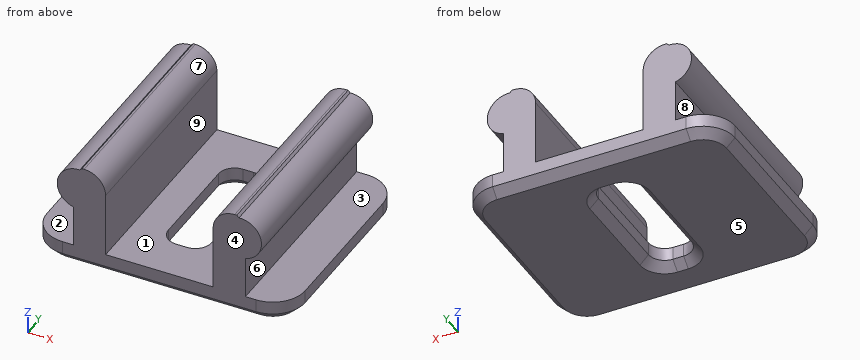
from build123d import *

# Parameters (mm, degrees)
BOX010_W                    = 2
BOX010_H                    = 6
BOX010_DEPTH                = 10
BOX008_W                    = 1.5
BOX008_H                    = 10
BOX008_DEPTH                = 5
CHAMFER004001002001005_SIZE = 0.4
CYLINDER004_R               = 1
CYLINDER004_DEPTH           = 10
CYLINDER003_R               = 1
CYLINDER003_DEPTH           = 10
BOX007_W                    = 12
BOX007_H                    = 10
BOX007_DEPTH                = 1
BOX009_W                    = 1.5
BOX009_H                    = 10
BOX009_DEPTH                = 5
CHAMFER004001002001006_SIZE = 0.4
FILLET_R                    = 0.75
FILLET001_R                 = 1.5
CHAMFER004001002001007_SIZE = 0.4
FILLET002_R                 = 1


with BuildPart() as cube010:
    # Box010 → Box010 (new body)
    with BuildSketch(Plane(origin=(-1, -3, 0), x_dir=(1, 0, 0), z_dir=(0, 0, 1))):
        with Locations((1, 3)):
            Rectangle(BOX010_W, BOX010_H)
    extrude(amount=BOX010_DEPTH)


with BuildPart() as chamfer004001002001005:
    # Box008 → Box008 (new body)
    with BuildSketch(Plane(origin=(-4, -5, 0), x_dir=(1, 0, 0), z_dir=(0, 0, 1))):
        with Locations((0.75, 5)):
            Rectangle(BOX008_W, BOX008_H)
    extrude(amount=BOX008_DEPTH)

    # Chamfer004001002001005
    chamfer004001002001005_edges = [chamfer004001002001005.edges().sort_by_distance(p)[0] for p in [
        (-4, 0, 5),
    ]]
    chamfer(chamfer004001002001005_edges, length=CHAMFER004001002001005_SIZE)


with BuildPart() as cylinder004:
    # Cylinder004 → Cylinder004 (new body)
    with BuildSketch(Plane(origin=(3.75, -5, 3.9), x_dir=(1, 0, 0), z_dir=(0, 1, 0))):
        Circle(CYLINDER004_R)
    extrude(amount=CYLINDER004_DEPTH)


with BuildPart() as cylinder003:
    # Cylinder003 → Cylinder003 (new body)
    with BuildSketch(Plane(origin=(-3.75, -5, 3.9), x_dir=(1, 0, 0), z_dir=(0, 1, 0))):
        Circle(CYLINDER003_R)
    extrude(amount=CYLINDER003_DEPTH)


with BuildPart() as cube007:
    # Box007 → Box007 (new body)
    with BuildSketch(Plane(origin=(-6, -5, 0), x_dir=(1, 0, 0), z_dir=(0, 0, 1))):
        with Locations((6, 5)):
            Rectangle(BOX007_W, BOX007_H)
    extrude(amount=BOX007_DEPTH)


with BuildPart() as cable_clip:
    # Box009 → Box009 (new body)
    with BuildSketch(Plane(origin=(2.5, -5, 0), x_dir=(1, 0, 0), z_dir=(0, 0, 1))):
        with Locations((0.75, 5)):
            Rectangle(BOX009_W, BOX009_H)
    extrude(amount=BOX009_DEPTH)

    # Chamfer004001002001006
    chamfer004001002001006_edges = [cable_clip.edges().sort_by_distance(p)[0] for p in [
        (4, 0, 5),
    ]]
    chamfer(chamfer004001002001006_edges, length=CHAMFER004001002001006_SIZE)

    # Fusion002: union Chamfer004001002001005, Cylinder004, Cylinder003, Cube007
    add(chamfer004001002001005.part)
    add(cylinder004.part)
    add(cylinder003.part)
    add(cube007.part)

    # Cut002008023012009006003002007003001002002: cut Cube010
    add(cube010.part, mode=Mode.SUBTRACT)

    # Fillet
    fillet_edges = [cable_clip.edges().sort_by_distance(p)[0] for p in [
        (1, -3, 0.5),
        (-1, -3, 0.5),
        (1, 3, 0.5),
        (-1, 3, 0.5),
    ]]
    fillet(fillet_edges, radius=FILLET_R)

    # Fillet001
    fillet001_edges = [cable_clip.edges().sort_by_distance(p)[0] for p in [
        (6, 5, 0.5),
        (-6, 5, 0.5),
        (6, -5, 0.5),
        (-6, -5, 0.5),
    ]]
    fillet(fillet001_edges, radius=FILLET001_R)

    # Chamfer004001002001007
    chamfer004001002001007_edges = [cable_clip.edges().sort_by_distance(p)[0] for p in [
        (4.25, -5, 0),
        (5.56066, -4.56066, 0),
        (6, 0, 0),
        (5.56066, 4.56066, 0),
        (3.25, 5, 0),
        (3.25, -5, 0),
        (0, 5, 0),
        (-1, 0, 0),
        (-0.78033, 2.78033, 0),
        (0, 3, 0),
        (0.78033, 2.78033, 0),
        (1, 0, 0),
        (0.78033, -2.78033, 0),
        (0, -3, 0),
        (-0.78033, -2.78033, 0),
        (0, -5, 0),
        (-3.25, 5, 0),
        (-3.25, -5, 0),
        (-4.25, 5, 0),
        (-5.56066, 4.56066, 0),
        (-6, 0, 0),
        (-5.56066, -4.56066, 0),
        (-4.25, -5, 0),
    ]]
    chamfer(chamfer004001002001007_edges, length=CHAMFER004001002001007_SIZE)

    # Fillet002
    fillet002_edges = [cable_clip.edges().sort_by_distance(p)[0] for p in [
        (2.5, 0, 5),
        (-2.5, 0, 5),
    ]]
    fillet(fillet002_edges, radius=FILLET002_R)


solid = cable_clip.part
Design review of the part built by this model. Coordinates are the model's own, in mm. Face numbers are marked on the shaded views. A direction names the side the tool comes from. Coordinates: 2 decimals unless noted, no trailing zeros. Order: outer loops, then holes, each group sorted by start corner. A loop starts at its lowest first (then second) coordinate and runs counter-clockwise, first axis right, second up. Notation, with made-up numbers: (74.25, 19) -> (125.25, 19) arc R12 cw to (125.25, 39) -> close; hole circle Ø10 at (71.5, 37). An arc over 180 degrees is marked (long way). One line per item, written item: value.
1) We need section A-A, the plane y = 2. Give the boundary of the cut face in (x, z), then the cut area to 3 significant figures.
Output values:
outline: (-6, 0.4) -> (-5.6, 0) -> (-1.4, 0) -> (-1, 0.4) -> (-1, 1) -> (-2.5, 1) -> (-2.5, 4) arc R1 ccw to (-3.5, 5) -> (-3.6, 5) -> (-3.7, 4.9) arc R1 ccw to (-4, 2.93) -> (-4, 1) -> (-6, 1) -> close; (1, 0.4) -> (1.4, 0) -> (5.6, 0) -> (6, 0.4) -> (6, 1) -> (4, 1) -> (4, 2.93) arc R1 ccw to (3.7, 4.9) -> (3.6, 5) -> (3.5, 5) arc R1 ccw to (2.5, 4) -> (2.5, 1) -> (1, 1) -> close
area: 23.3 mm2
2) Machinability: for the marked faces 1, 2, 3, 4 and 5, which of the approach directions +Z, -Z, +X, -X, +Y, -Y give a long, thin tool a straight path to every point of the face, cutting with its end or side? Answer none if there is none.
Output values:
face 1: +Z, +Y, -Y
face 2: -X, +Y, -Y
face 3: +X, +Y, -Y
face 4: +Z, -Z, +X, -X, -Y
face 5: -Z, +X, -X, +Y, -Y
3) Draft analysis for pull direction Z (two halves, no side actions). For the marked faces 6, 7, 8 and 9, state which applies: +Z half, -Z half, draft (parallel to the pull), parting line (faces both ways), or undercut.
Output values:
face 6: undercut
face 7: +Z half
face 8: undercut
face 9: draft
4) Clearance check with flat-ended pins moving along their axes: P1, Ø3, axis at x = 2.5, z = 4.5, coming from the -Y side; P2, Ø2, axis at y = 2.5, z = 3, coming from the +X side; P3, Ø1, axis at y = 2, z = 2, coming from the -X side; P4, Ø2, axis at x = -5.5, y = -2, coming from the +Z side. State where each tip first meets the part, or that it passes through.
Output values:
P1: stops at y = -5
P2: stops at x = 4.75
P3: stops at x = -4
P4: stops at z = 4.56
5) We need section B-B, the plane z = 2.2. Give the boundary of the cut face in (x, y).
Output values:
outline: (-4, -5) -> (-2.5, -5) -> (-2.5, 5) -> (-4, 5) -> close; (2.5, -5) -> (4, -5) -> (4, 5) -> (2.5, 5) -> close
6) We need section D-D, the plane z = 3.45. Give the boundary of the cut face in (x, y), then the cut area to 3 significant figures.
Output values:
outline: (-4.64, -5) -> (-2.5, -5) -> (-2.5, 5) -> (-4.64, 5) -> close; (2.5, -5) -> (4.64, -5) -> (4.64, 5) -> (2.5, 5) -> close
area: 42.9 mm2
7) To check wall thickness, follow probe 1 along X at (y, z) = (2, 1.55); probe 2 along Y at (x, z) = (0, 0.8); probe 3 along Z at (x, y) = (-2, 2). State the ranges of each line that lie inside material, in increasing order. Write a range as [from, to].
Output values:
probe 1: x = [-4, -2.5], [2.5, 4]
probe 2: y = [-5, -3], [3, 5]
probe 3: z = [0, 1]
8) We need section C-C, the plane x = -1.75. Give the boundary of the cut face in (y, z).
Output values:
outline: (-5, 0.4) -> (-4.6, 0) -> (4.6, 0) -> (5, 0.4) -> (5, 1) -> (-5, 1) -> close
